Could you check a few things on this model? Use its own coordinates, in mm. A direction names the side the tool comes from. Round coordinates to 2 decimals unless told otherwise and drop trailing zeros. Loops run counter-clockwise (first coordinate to the right, second up) from the corner with the lowest first, then second, coordinate; pieces in that order, holes last. Notation, with made-up numbers: (-31.5, 40) - (-13.5, 40) arc R22 ccw to (-13.5, 57) - close; hole circle Ø9 at (-40, 44). An arc over 180 degrees is marked (long way). Use one line per item in the form item = value.
```python
from build123d import *

# Parameters (mm, degrees)
SKETCH1_W           = 20
SKETCH1_H           = 220
BOSS_EXTRUDE1_DEPTH = 20
SKETCH2_W           = 60
SKETCH2_H           = 20
BOSS_EXTRUDE2_DEPTH = 30
SKETCH3_W           = 70
SKETCH3_H           = 30
SKETCH3_W_2         = 60
SKETCH3_H_2         = 20
BOSS_EXTRUDE3_DEPTH = 10
FILLET1_R           = 1
FILLET2_R           = 1


with BuildPart() as part:
    # Sketch1 → Boss-Extrude1 (new body)
    with BuildSketch(Plane.XY):
        with BuildLine():
            Line((30, 0), (30, -100))
            Line((30, -100), (40, -100))
            Line((40, -100), (40, -160))
            Line((40, -160), (30, -160))
            Line((30, -160), (30, -260))
            ThreePointArc((30, -260), (0, -290), (-30, -260))
            Line((-30, -260), (-30, -160))
            Line((-30, -160), (-40, -160))
            Line((-40, -160), (-40, -100))
            Line((-40, -100), (-30, -100))
            Line((-30, -100), (-30, 0))
            ThreePointArc((-30, 0), (0, 30), (30, 0))
        make_face()
        with Locations((0, -130)):
            Rectangle(SKETCH1_W, SKETCH1_H, mode=Mode.SUBTRACT)
    extrude(amount=BOSS_EXTRUDE1_DEPTH)

    # Sketch2 → Boss-Extrude2 (add)
    with BuildSketch(Plane.XY.offset(20)):
        with Locations((0, -130)):
            Rectangle(SKETCH2_W, SKETCH2_H)
    extrude(amount=BOSS_EXTRUDE2_DEPTH)

    # Sketch3 → Boss-Extrude3 (add)
    with BuildSketch(Plane.XY.offset(20)):
        with Locations((0, -130)):
            Rectangle(SKETCH3_W, SKETCH3_H)
        with Locations((0, -130)):
            Rectangle(SKETCH3_W_2, SKETCH3_H_2, mode=Mode.SUBTRACT)
    extrude(amount=BOSS_EXTRUDE3_DEPTH)

    # Fillet1
    fillet1_edges = [part.edges().sort_by_distance(p)[0] for p in [
        (-30, -130, 50),
        (0, -140, 50),
        (30, -130, 50),
        (0, -120, 50),
        (35, -130, 30),
        (0, -115, 30),
        (-35, -130, 30),
        (0, -145, 30),
        (0, -120, 30),
        (-30, -130, 30),
        (0, -140, 30),
        (30, -130, 30),
    ]]
    fillet(fillet1_edges, radius=FILLET1_R)

    # Fillet2
    fillet2_edges = [part.edges().sort_by_distance(p)[0] for p in [
        (30, -50, 0),
        (35, -100, 0),
        (-35, -100, 20),
        (40, -130, 0),
        (35, -160, 0),
        (30, -210, 0),
        (0, -290, 0),
        (-30, -210, 0),
        (-35, -160, 0),
        (-40, -130, 0),
        (-35, -100, 0),
        (-30, -50, 0),
        (0, 30, 0),
        (-40, -130, 20),
        (-35, -160, 20),
        (-30, -210, 20),
        (0, -290, 20),
        (30, -210, 20),
        (35, -160, 20),
        (40, -130, 20),
        (35, -100, 20),
        (30, -50, 20),
        (0, 30, 20),
        (-30, -50, 20),
    ]]
    fillet(fillet2_edges, radius=FILLET2_R)


solid = part.part
```
1. If we section it at A-A, the plane y = -73.5: Write out the boundary of the cut face in (x, z), plus the area to 3 significant figures.
Solution:
outline = (-30, 1) arc R1 ccw to (-29, 0) - (-10, 0) - (-10, 20) - (-29, 20) arc R1 ccw to (-30, 19) - close; (10, 0) - (29, 0) arc R1 ccw to (30, 1) - (30, 19) arc R1 ccw to (29, 20) - (10, 20) - close
area = 799 mm^2
2. On a 3-axis mill with a long thin cutter (end or side, diameter ignored), from which of +Z, -Z, +X, -X, +Y, -Y can I reach the whole of each face in a straight line? I mean faces 1 (the face through (-30, -51, 10)), 2 (the face through (-35, -130, 24)), 3 (the face through (0, -120, 40)), 4 (the face through (0, -145, 24)). Say none if no direction works.
Solution:
face_1 = +Z, -Z, -X, +Y
face_2 = +Z, -X, +Y, -Y
face_3 = +Z, +X, -X, +Y
face_4 = +Z, +X, -X, -Y
3. Please list where these lines run through material, in increasing order: line 1 along X through (y, z) = (-54, 3.5); line 2 along Z through (x, y) = (26, -88.5); line 3 along X through (y, z) = (-4, 6.5).
Solution:
line_1 = -30 to -10, 10 to 30
line_2 = 0 to 20
line_3 = -30 to 30
4. If we section it at B-B, the plane z = 9: Write out the boundary of the cut face in (x, y), plus the area to 3 significant figures.
Solution:
outline = (-40, -160) - (-30, -160) - (-30, -260) arc R30 ccw to (30, -260) - (30, -160) - (40, -160) - (40, -100) - (30, -100) - (30, 0) arc R30 ccw to (-30, 0) - (-30, -100) - (-40, -100) - close; hole (-10, -240) - (10, -240) - (10, -20) - (-10, -20) - close
area = 15,200 mm^2
5. For P1, Ø20, axis at y = -38, z = 11.5, coming from the +X side; P2, Ø5, axis at x = 34, z = 6, coming from the -Y side; P3, Ø3, axis at x = 36, z = 10.5, coming from the +Y side; P4, Ø10, axis at y = -150.5, z = 34, coming from the +X side, each with a flat end and sliding along its axis, tell me the tip position at first contact or that it passes through.
Solution:
P1 = 30
P2 = -160
P3 = -100
P4 = through
6. We'd pull the mould along X, two halves only. Please class faces 5 (the face through (0.66, -289.993, 9.874)), 6 (the face through (0, -20, 10)), 7 (the face through (35, -100, 10)), 8 (the face through (0, -240, 10)): +X half, -X half, draft (parallel to the pull), parting line (faces both ways), or undercut.
Solution:
face_5 = parting line
face_6 = undercut
face_7 = draft
face_8 = undercut
7. If we section it at C-C, the plane x = 0: Write out the boundary of the cut face in (y, z), plus the area to 3 significant figures.
Solution:
outline = (-290, 1) arc R1 ccw to (-289, 0) - (-240, 0) - (-240, 20) - (-289, 20) arc R1 ccw to (-290, 19) - close; (-145, 20) - (-115, 20) - (-115, 29) arc R1 ccw to (-116, 30) - (-119, 30) arc R1 cw to (-120, 31) - (-120, 49) arc R1 ccw to (-121, 50) - (-139, 50) arc R1 ccw to (-140, 49) - (-140, 31) arc R1 cw to (-141, 30) - (-144, 30) arc R1 ccw to (-145, 29) - close; (-20, 0) - (29, 0) arc R1 ccw to (30, 1) - (30, 19) arc R1 ccw to (29, 20) - (-20, 20) - close
area = 2,700 mm^2
8. If we section it at D-D, the plane z = 35.5: Write out the boundary of the cut face in (x, y), plus the area to 3 significant figures.
Solution:
outline = (-30, -140) - (30, -140) - (30, -120) - (-30, -120) - close
area = 1,200 mm^2
